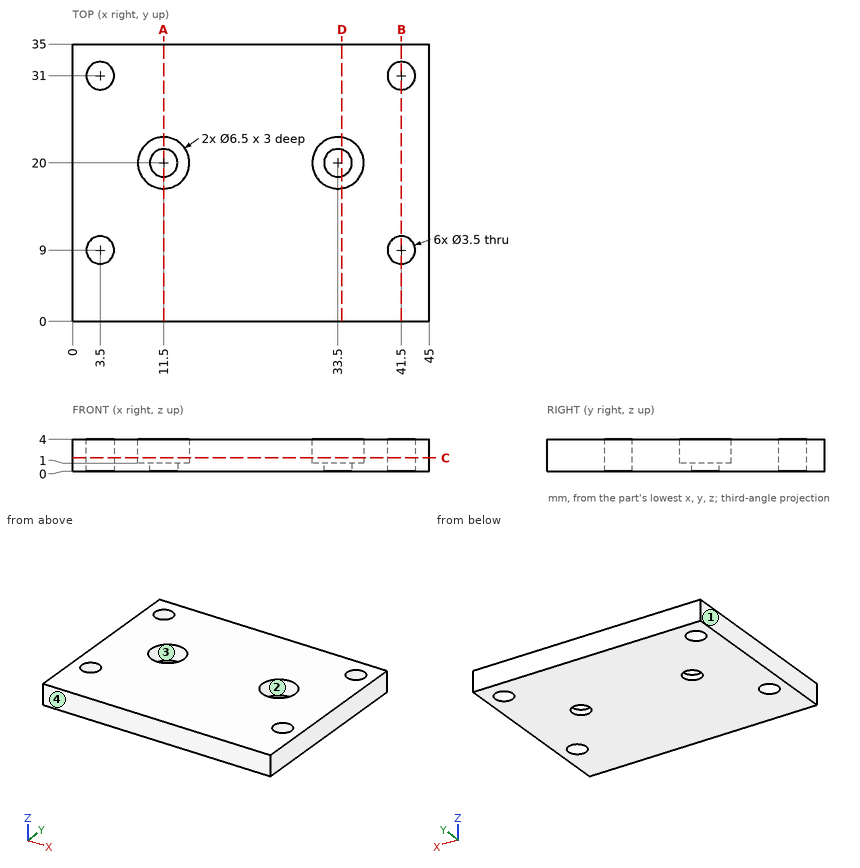
Study the drawing (mm; zero at the part's minimum x, y, z) and answer. Give positions to 0.01 mm unless a question says otherwise; leave off trailing zeros. Order: outer loops, then holes, each group sorted by start corner. A loop starts at its lowest first (then second) coordinate and runs counter-clockwise, first axis right, second up. Notation, with made-up numbers: (20, 16) - (76, 16) arc R18 ccw to (76, 22) - close; hole circle Ø4 at (73, 13.5). An arc over 180 degrees is marked (long way). Answer in a Markdown table with one row per item. Add a question column.
Q1. Find the intervals of material crossed by line 1 along Y through (x, z) = (33.5, 2.45); line 2 along Y through (x, z) = (4, 1.3); line 3 along X through (y, z) = (23, 3), in increasing order. Write a range as [from, to].
Q2. The part is cut by section C-C (z = 1.65). Determine the outline of the cut face in (x, y), then the cut area to 3 significant figures.
Q3. Given P1, Ø5.5, axis at x = 3.5, y = 31, coming from the -Z side; P2, Ø3, axis at x = 33.5, y = 21.5, coming from the +Z side, each flat-ended and moving along its own axis, determine where each tip first touches the part or whether it passes through.
Q4. The part is cut by section B-B (x = 41.5). Determine the outline of the cut face in (y, z), then the cut area to 3 significant figures.
Q5. The part is cut by section A-A (x = 11.5). Determine the outline of the cut face in (y, z), then the cut area to 3 significant figures.
Q6. The part is cut by section D-D (x = 34). Determine the outline of the cut face in (y, z), then the cut area to 3 significant figures.
Q7. For a pull along X with two mould halves and no side action, classify the marked faces 1, 2, 3 and 4 as released by +X, released by -X, zero draft, split by the parting line, or undercut.
Determined:
| question | item | result |
|---|---|---|
| 1 | line 1 | y = [0, 16.75], [23.25, 35] |
| 1 | line 2 | y = [0, 7.32], [10.68, 29.32], [32.68, 35] |
| 1 | line 3 | x = [0, 10.25], [12.75, 32.25], [34.75, 45] |
| 2 | outline | (0, 0) - (45, 0) - (45, 35) - (0, 35) - close; hole circle Ø3.5 at (3.5, 9); hole circle Ø3.5 at (3.5, 31); hole circle Ø6.5 at (11.5, 20); hole circle Ø6.5 at (33.5, 20); hole circle Ø3.5 at (41.5, 9); hole circle Ø3.5 at (41.5, 31) |
| 2 | area | 1,470 mm² |
| 3 | P1 | stops at z = 0 |
| 3 | P2 | stops at z = 1 |
| 4 | outline | (0, 0) - (7.25, 0) - (7.25, 4) - (0, 4) - close; (10.75, 0) - (29.25, 0) - (29.25, 4) - (10.75, 4) - close; (32.75, 0) - (35, 0) - (35, 4) - (32.75, 4) - close |
| 4 | area | 112 mm² |
| 5 | outline | (0, 0) - (18.25, 0) - (18.25, 1) - (16.75, 1) - (16.75, 4) - (0, 4) - close; (21.75, 0) - (35, 0) - (35, 4) - (23.25, 4) - (23.25, 1) - (21.75, 1) - close |
| 5 | area | 117 mm² |
| 6 | outline | (0, 0) - (18.32, 0) - (18.32, 1) - (16.79, 1) - (16.79, 4) - (0, 4) - close; (21.68, 0) - (35, 0) - (35, 4) - (23.21, 4) - (23.21, 1) - (21.68, 1) - close |
| 6 | area | 117 mm² |
| 7 | face 1 | released by -X |
| 7 | face 2 | undercut |
| 7 | face 3 | undercut |
| 7 | face 4 | zero draft |
